Read the model definition and answer for the solid it produces. Units are mm, in the model's axes. A direction names the side the tool comes from. Give positions to 0.01 mm unless a question says otherwise; leave off trailing zeros. Write each loop counter-clockwise with the first axis right and the second up, starting at its lowest first coordinate (ties: lowest second). Pieces come first, ordered by that corner, then holes. Notation, with made-up numbers: M 85,77 L 126,77 A9 cw 126,90 Z; hole C 64.25,75.5 d1. An arc over 180 degrees is marked long. Use a Markdown table: item, result. Add a question column.
Item 1: A cutting plane is placed at A-A on y = 0. Determine the outline of the cut face in (x, z).
Item 2: Given P1, Ø2, axis at y = 0, z = 1, coming from the +X side; P2, Ø3, axis at x = 0, y = 0, coming from the +Z side; P3, Ø1.5, axis at x = 0, y = 0, coming from the +Z side, each flat-ended and moving along its own axis, determine where each tip first touches the part or whether it passes through.
Item 3: For faces 1 (the flat face through (4.38, -0.91, 1.52)), 2 (the flat face through (2.1, -2.2, 3)), 3 (the flat face through (-4.39, 0.94, 1.52)), determine the directions among +Z, -Z, +X, -X, +Y, -Y from which every point of the face is accessible in a straight line to the end or side of a thin tool.
Item 4: Consider probe 1 along X at (y, z) = (0, -1); probe 2 along X at (y, z) = (2.75, 0.5). Determine where each line is inside the solid, lowest interval first. Write a range as [from, to].
Item 5: A cutting plane is placed at B-B on z = -0.7. Determine the outline of the cut face in (x, y), then the cut area to 3 significant figures.
Item 6: A cutting plane is placed at D-D on y = 4.25. Determine the outline of the cut face in (x, z), then the cut area to 3 significant figures.
Item 7: A cutting plane is placed at C-C on y = -3. Determine the outline of the cut face in (x, z).
Item 8: The mould has two halves that part along X. Classify faces 4 (the flat face through (4.5, 0, 1.5)), 5 (the flat face through (-4.096, 1.804, 1.521)), 6 (the flat face through (0.485, -4.449, 1.521)), 7 (the flat face through (0, 1, 0.9)): pulls with the +X half, pulls with the -X half, needs draft (parallel to the pull), parting line crosses it, or undercut.
from build123d import *

# Parameters (mm, degrees)
SKETCH_R           = 5
PAD_DEPTH          = 3
SKETCH001_R        = 2.8
PAD001_DEPTH       = 0.9
SKETCH002_R        = 1.8
POCKET_DEPTH       = 1.1
SKETCH003_R        = 3.2
PAD002_DEPTH       = 1.7
SKETCH004_R        = 2.3
POCKET001_DEPTH    = 2.6
SKETCH005_R        = 0.4
POCKET002_DEPTH    = 4.701
POCKET003_DEPTH    = 35.122045
POLARPATTERN_COUNT = 15
SKETCH008_R        = 0.85
POCKET004_DEPTH    = 4.501


with BuildPart() as part:
    # Sketch → Pad (new body)
    with BuildSketch(Plane.XY):
        Circle(SKETCH_R)
    extrude(amount=PAD_DEPTH)

    # Sketch001 → Pad001 (new body)
    with BuildSketch(Plane.XY.offset(3)):
        Circle(SKETCH001_R)
    extrude(amount=PAD001_DEPTH)

    # Sketch002 → Pocket (cut)
    with BuildSketch(Plane.XY.offset(3.9)):
        Circle(SKETCH002_R)
    extrude(amount=-POCKET_DEPTH, mode=Mode.SUBTRACT)

    # Sketch003 → Pad002 (new body)
    with BuildSketch(Plane(origin=(0, 0, 0), x_dir=(1, 0, 0), z_dir=(0, 0, -1))):
        Circle(SKETCH003_R)
    extrude(amount=PAD002_DEPTH)

    # Sketch004 → Pocket001 (cut)
    with BuildSketch(Plane(origin=(0, 0, -1.7), x_dir=(1, 0, 0), z_dir=(0, 0, -1))):
        Circle(SKETCH004_R)
    extrude(amount=-POCKET001_DEPTH, mode=Mode.SUBTRACT)

    # Sketch005 → Pocket002 (cut, through all)
    with BuildSketch(Plane.XY.offset(3)):
        with Locations((-1.8, 7.126184)):
            Circle(SKETCH005_R)
        with Locations((1.8, 7.126184)):
            Circle(SKETCH005_R)
    extrude(amount=-POCKET002_DEPTH, mode=Mode.SUBTRACT)

    # Sketch007 → Pocket003 (cut, through all)
    with BuildSketch(Plane.XY.offset(3)):
        Polygon((-1, 5.002483), (0, 4.002483), (1, 5.002483), align=None)
    pocket003 = extrude(amount=-POCKET003_DEPTH, mode=Mode.SUBTRACT)

    # PolarPattern: Pocket003 ×15 about axis
    polarpattern_axis = Axis((0, 0, 3), (0, 0, 1))
    for i in range(1, POLARPATTERN_COUNT):
        add(pocket003.rotate(polarpattern_axis, i * 360 / POLARPATTERN_COUNT), mode=Mode.SUBTRACT)

    # Sketch008 → Pocket004 (cut, through all)
    with BuildSketch(Plane.XY.offset(2.8)):
        Circle(SKETCH008_R)
    extrude(amount=-POCKET004_DEPTH, mode=Mode.SUBTRACT)


solid = part.part
Filled in:
| question | item | result |
|---|---|---|
| 1 | outline | M -4.5,0 L -3.2,0 L -3.2,-1.7 L -2.3,-1.7 L -2.3,0.9 L -0.85,0.9 L -0.85,2.8 L -1.8,2.8 L -1.8,3.9 L -2.8,3.9 L -2.8,3 L -4.5,3 Z; M 0.85,0.9 L 2.3,0.9 L 2.3,-1.7 L 3.2,-1.7 L 3.2,0 L 4.5,0 L 4.5,3 L 2.8,3 L 2.8,3.9 L 1.8,3.9 L 1.8,2.8 L 0.85,2.8 Z |
| 2 | P1 | x = 4.98 |
| 2 | P2 | z = 2.8 |
| 2 | P3 | through |
| 3 | face 1 | +Z, -Z, +X |
| 3 | face 2 | +Z |
| 3 | face 3 | +Z, -Z, -X |
| 4 | probe 1 | [-3.2, -2.3], [2.3, 3.2] |
| 4 | probe 2 | [-2.98, 2.98] |
| 5 | outline | C 0,0 d6.4; hole C 0,0 d4.6 |
| 5 | area | 15.6 mm² |
| 6 | outline | M -1.4,0 L -0.25,0 L -0.25,3 L -1.4,3 Z; M 0.25,0 L 1.4,0 L 1.4,3 L 0.25,3 Z |
| 6 | area | 6.92 mm² |
| 7 | outline | M -3.73,0 L -1.11,0 L -1.11,-1.7 L 1.11,-1.7 L 1.11,0 L 3.73,0 L 3.73,3 L -3.73,3 Z |
| 8 | face 4 | pulls with the +X half |
| 8 | face 5 | pulls with the -X half |
| 8 | face 6 | undercut |
| 8 | face 7 | undercut |
